Input: part model. Units: mm. Frame: model coordinates. Face numbers are marked on the shaded views. A direction names the side the tool comes from. Give positions to 0.01 mm unless a question says otherwise; leave off trailing zeros. Write each loop counter-clockwise with the first axis right and the second up, starting at its lowest first coordinate (ties: lowest second). Pieces come first, ordered by that corner, then holes. Notation, with made-up numbers: (55.5, -6.5) -> (100.5, -6.5) arc R29 cw to (100.5, 15.5) -> close; hole circle Ø5 at (-28, 54). An arc over 180 degrees is marked (long way). Return JSON: item names as keys, results as strings. Group by question number.
Item 1: Mould query, pull axis X, two halves, no side actions, for the marked faces 4, 5, 6 and 7. Classes: released by +X, released by -X, zero draft, split by the parting line, or undercut.
Item 2: Section D-D, the plane y = 21.5. Return loops of the section in (x, z).
Item 3: Pin query (flat end, axial travel): P1, Ø3, axis at x = 88, y = 47.5, coming from the +Z side; P2, Ø4, axis at x = 31.5, y = 11, coming from the +Z side. Return the tip coordinate at first contact, or that it passes through.
Item 4: Section B-B, the plane z = 8.5. Return loops of the section in (x, y).
Item 5: Section A-A, the plane y = 81.75. Return loops of the section in (x, z).
Item 6: Line query: line 1 (Y direction, x = 139.5, z = 19.5); line 2 (X direction, y = 5.75, z = 26); line 3 (Z direction, x = 146, y = 36). Output: solid intervals per line, ascending. Write a range as [from, to].
Item 7: Set-up query: the marked faces 1, 2 and 3. Return all of +Z, -Z, +X, -X, +Y, -Y with unobstructed straight access to the full face (end or side cutting, diameter ignored); none if empty.
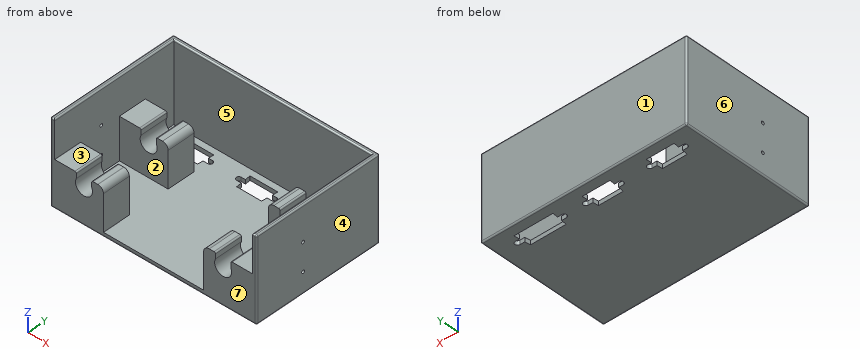
from build123d import *

# Parameters (mm, degrees)
CYLINDER009_R      = 1.1
CYLINDER009_DEPTH  = 150
CYLINDER008_R      = 1.1
CYLINDER008_DEPTH  = 150
BOX011_W           = 25.4
BOX011_H           = 3.6
BOX011_DEPTH       = 10
CYLINDER005_R      = 1.8
CYLINDER005_DEPTH  = 10
CYLINDER004_R      = 1.8
CYLINDER004_DEPTH  = 10
BOX010_W           = 20
BOX010_H           = 11.5
BOX010_DEPTH       = 10
CHAMFER001_1_SIZE2 = 1.1
CHAMFER001_1_SIZE  = 11
CHAMFER001_2_SIZE2 = 1.1
CHAMFER001_2_SIZE  = 11
BOX013_W           = 25.4
BOX013_H           = 3.6
BOX013_DEPTH       = 10
CYLINDER006_R      = 1.8
CYLINDER006_DEPTH  = 10
CYLINDER007_R      = 1.8
CYLINDER007_DEPTH  = 10
BOX012_W           = 20
BOX012_H           = 11.5
BOX012_DEPTH       = 10
CHAMFER002_1_SIZE2 = 1.1
CHAMFER002_1_SIZE  = 11
CHAMFER002_2_SIZE2 = 1.1
CHAMFER002_2_SIZE  = 11
CYLINDER003_R      = 1.8
CYLINDER003_DEPTH  = 10
BOX009_W           = 33.6
BOX009_H           = 3.6
BOX009_DEPTH       = 10
CYLINDER002_R      = 1.8
CYLINDER002_DEPTH  = 10
BOX008_W           = 28
BOX008_H           = 11.5
BOX008_DEPTH       = 10
CHAMFER_1_SIZE2    = 1.2
CHAMFER_1_SIZE     = 11
CHAMFER_2_SIZE2    = 1.2
CHAMFER_2_SIZE     = 11
BOX006_W           = 11
BOX006_H           = 73
BOX006_DEPTH       = 15
BOX007_W           = 11
BOX007_H           = 73
BOX007_DEPTH       = 15
CYLINDER001_R      = 6.1
CYLINDER001_DEPTH  = 80
CYLINDER_R         = 6.1
CYLINDER_DEPTH     = 80
BOX002_W           = 35
BOX002_H           = 20
BOX002_DEPTH       = 30
BOX003_W           = 35
BOX003_H           = 20
BOX003_DEPTH       = 30
BOX004_W           = 35
BOX004_H           = 20
BOX004_DEPTH       = 30
BOX005_W           = 35
BOX005_H           = 20
BOX005_DEPTH       = 30
BOX001_W           = 142
BOX001_H           = 92
BOX001_DEPTH       = 60
BOX_W              = 148
BOX_H              = 95
BOX_DEPTH          = 60
FILLET_R           = 1
FILLET001_R        = 4
FILLET002_R        = 1


with BuildPart() as cylinder009:
    # Cylinder009 → Cylinder009 (new body)
    with BuildSketch(Plane(origin=(-1, 36, 35), x_dir=(0, 0, -1), z_dir=(1, 0, 0))):
        Circle(CYLINDER009_R)
    extrude(amount=CYLINDER009_DEPTH)


with BuildPart() as cylinder008:
    # Cylinder008 → Cylinder008 (new body)
    with BuildSketch(Plane(origin=(-1, 36, 15), x_dir=(0, 0, -1), z_dir=(1, 0, 0))):
        Circle(CYLINDER008_R)
    extrude(amount=CYLINDER008_DEPTH)


with BuildPart() as cube011:
    # Box011 → Box011 (new body)
    with BuildSketch(Plane(origin=(-2.7, 3.95, 0), x_dir=(1, 0, 0), z_dir=(0, 0, 1))):
        with Locations((12.7, 1.8)):
            Rectangle(BOX011_W, BOX011_H)
    extrude(amount=BOX011_DEPTH)


with BuildPart() as cylinder005:
    # Cylinder005 → Cylinder005 (new body)
    with BuildSketch(Plane(origin=(22.7, 5.75, 0), x_dir=(1, 0, 0), z_dir=(0, 0, 1))):
        Circle(CYLINDER005_R)
    extrude(amount=CYLINDER005_DEPTH)


with BuildPart() as cylinder004:
    # Cylinder004 → Cylinder004 (new body)
    with BuildSketch(Plane(origin=(-2.7, 5.75, 0), x_dir=(1, 0, 0), z_dir=(0, 0, 1))):
        Circle(CYLINDER004_R)
    extrude(amount=CYLINDER004_DEPTH)


with BuildPart() as obj1:
    # Box010 → Box010 (new body)
    with BuildSketch(Plane.XY):
        with Locations((10, 5.75)):
            Rectangle(BOX010_W, BOX010_H)
    extrude(amount=BOX010_DEPTH)

    # Chamfer001 1
    chamfer001_1_edges = [obj1.edges().sort_by_distance(p)[0] for p in [
        (20, 0, 5),
    ]]
    chamfer001_1_side = obj1.faces().sort_by_distance((20, 5.75, 5))[0]
    chamfer(chamfer001_1_edges, length=CHAMFER001_1_SIZE, length2=CHAMFER001_1_SIZE2, reference=chamfer001_1_side)

    # Chamfer001 2
    chamfer001_2_edges = [obj1.edges().sort_by_distance(p)[0] for p in [
        (0, 0, 5),
    ]]
    chamfer001_2_side = obj1.faces().sort_by_distance((0, 5.75, 5))[0]
    chamfer(chamfer001_2_edges, length=CHAMFER001_2_SIZE, length2=CHAMFER001_2_SIZE2, reference=chamfer001_2_side)

    # Fusion002: union Cube011, Cylinder005, Cylinder004
    add(cube011.part)
    add(cylinder005.part)
    add(cylinder004.part)


with BuildPart() as obj1_1:
    # Fusion002 placement: moved
    add(obj1.part.moved(Location((16, 76, 0))))


with BuildPart() as cube013:
    # Box013 → Box013 (new body)
    with BuildSketch(Plane(origin=(-2.7, 3.95, 0), x_dir=(1, 0, 0), z_dir=(0, 0, 1))):
        with Locations((12.7, 1.8)):
            Rectangle(BOX013_W, BOX013_H)
    extrude(amount=BOX013_DEPTH)


with BuildPart() as cylinder006:
    # Cylinder006 → Cylinder006 (new body)
    with BuildSketch(Plane(origin=(22.7, 5.75, 0), x_dir=(1, 0, 0), z_dir=(0, 0, 1))):
        Circle(CYLINDER006_R)
    extrude(amount=CYLINDER006_DEPTH)


with BuildPart() as cylinder007:
    # Cylinder007 → Cylinder007 (new body)
    with BuildSketch(Plane(origin=(-2.7, 5.75, 0), x_dir=(1, 0, 0), z_dir=(0, 0, 1))):
        Circle(CYLINDER007_R)
    extrude(amount=CYLINDER007_DEPTH)


with BuildPart() as obj2:
    # Box012 → Box012 (new body)
    with BuildSketch(Plane.XY):
        with Locations((10, 5.75)):
            Rectangle(BOX012_W, BOX012_H)
    extrude(amount=BOX012_DEPTH)

    # Chamfer002 1
    chamfer002_1_edges = [obj2.edges().sort_by_distance(p)[0] for p in [
        (20, 0, 5),
    ]]
    chamfer002_1_side = obj2.faces().sort_by_distance((20, 5.75, 5))[0]
    chamfer(chamfer002_1_edges, length=CHAMFER002_1_SIZE, length2=CHAMFER002_1_SIZE2, reference=chamfer002_1_side)

    # Chamfer002 2
    chamfer002_2_edges = [obj2.edges().sort_by_distance(p)[0] for p in [
        (0, 0, 5),
    ]]
    chamfer002_2_side = obj2.faces().sort_by_distance((0, 5.75, 5))[0]
    chamfer(chamfer002_2_edges, length=CHAMFER002_2_SIZE, length2=CHAMFER002_2_SIZE2, reference=chamfer002_2_side)

    # Fusion003: union Cube013, Cylinder006, Cylinder007
    add(cube013.part)
    add(cylinder006.part)
    add(cylinder007.part)


with BuildPart() as obj2_1:
    # Fusion003 placement: moved
    add(obj2.part.moved(Location((62, 76, 0))))


with BuildPart() as cylinder003:
    # Cylinder003 → Cylinder003 (new body)
    with BuildSketch(Plane(origin=(30.8, 5.75, 0), x_dir=(1, 0, 0), z_dir=(0, 0, 1))):
        Circle(CYLINDER003_R)
    extrude(amount=CYLINDER003_DEPTH)


with BuildPart() as cube009:
    # Box009 → Box009 (new body)
    with BuildSketch(Plane(origin=(-2.8, 3.95, 0), x_dir=(1, 0, 0), z_dir=(0, 0, 1))):
        with Locations((16.8, 1.8)):
            Rectangle(BOX009_W, BOX009_H)
    extrude(amount=BOX009_DEPTH)


with BuildPart() as cylinder002:
    # Cylinder002 → Cylinder002 (new body)
    with BuildSketch(Plane(origin=(-2.8, 5.75, 0), x_dir=(1, 0, 0), z_dir=(0, 0, 1))):
        Circle(CYLINDER002_R)
    extrude(amount=CYLINDER002_DEPTH)


with BuildPart() as obj3:
    # Box008 → Box008 (new body)
    with BuildSketch(Plane.XY):
        with Locations((14, 5.75)):
            Rectangle(BOX008_W, BOX008_H)
    extrude(amount=BOX008_DEPTH)

    # Chamfer 1
    chamfer_1_edges = [obj3.edges().sort_by_distance(p)[0] for p in [
        (28, 0, 5),
    ]]
    chamfer_1_side = obj3.faces().sort_by_distance((28, 5.75, 5))[0]
    chamfer(chamfer_1_edges, length=CHAMFER_1_SIZE, length2=CHAMFER_1_SIZE2, reference=chamfer_1_side)

    # Chamfer 2
    chamfer_2_edges = [obj3.edges().sort_by_distance(p)[0] for p in [
        (0, 0, 5),
    ]]
    chamfer_2_side = obj3.faces().sort_by_distance((0, 5.75, 5))[0]
    chamfer(chamfer_2_edges, length=CHAMFER_2_SIZE, length2=CHAMFER_2_SIZE2, reference=chamfer_2_side)

    # Fusion001: union Cylinder003, Cube009, Cylinder002
    add(cylinder003.part)
    add(cube009.part)
    add(cylinder002.part)


with BuildPart() as obj3_1:
    # Fusion001 placement: moved
    add(obj3.part.moved(Location((103, 76, 0))))


with BuildPart() as cube006:
    # Box006 → Box006 (new body)
    with BuildSketch(Plane(origin=(118.5, 0, 27), x_dir=(1, 0, 0), z_dir=(0, 0, 1))):
        with Locations((5.5, 36.5)):
            Rectangle(BOX006_W, BOX006_H)
    extrude(amount=BOX006_DEPTH)


with BuildPart() as cube007:
    # Box007 → Box007 (new body)
    with BuildSketch(Plane(origin=(18.5, 0, 27), x_dir=(1, 0, 0), z_dir=(0, 0, 1))):
        with Locations((5.5, 36.5)):
            Rectangle(BOX007_W, BOX007_H)
    extrude(amount=BOX007_DEPTH)


with BuildPart() as cylinder001:
    # Cylinder001 → Cylinder001 (new body)
    with BuildSketch(Plane(origin=(124, 73, 26), x_dir=(1, 0, 0), z_dir=(0, -1, 0))):
        Circle(CYLINDER001_R)
    extrude(amount=CYLINDER001_DEPTH)


with BuildPart() as cylinder:
    # Cylinder → Cylinder (new body)
    with BuildSketch(Plane(origin=(24, 73, 26), x_dir=(1, 0, 0), z_dir=(0, -1, 0))):
        Circle(CYLINDER_R)
    extrude(amount=CYLINDER_DEPTH)


with BuildPart() as cube002:
    # Box002 → Box002 (new body)
    with BuildSketch(Plane(origin=(3, 0, 3), x_dir=(1, 0, 0), z_dir=(0, 0, 1))):
        with Locations((17.5, 10)):
            Rectangle(BOX002_W, BOX002_H)
    extrude(amount=BOX002_DEPTH)


with BuildPart() as cube003:
    # Box003 → Box003 (new body)
    with BuildSketch(Plane(origin=(3, 50, 3), x_dir=(1, 0, 0), z_dir=(0, 0, 1))):
        with Locations((17.5, 10)):
            Rectangle(BOX003_W, BOX003_H)
    extrude(amount=BOX003_DEPTH)


with BuildPart() as cube004:
    # Box004 → Box004 (new body)
    with BuildSketch(Plane(origin=(110, 0, 3), x_dir=(1, 0, 0), z_dir=(0, 0, 1))):
        with Locations((17.5, 10)):
            Rectangle(BOX004_W, BOX004_H)
    extrude(amount=BOX004_DEPTH)


with BuildPart() as cube005:
    # Box005 → Box005 (new body)
    with BuildSketch(Plane(origin=(110, 50, 3), x_dir=(1, 0, 0), z_dir=(0, 0, 1))):
        with Locations((17.5, 10)):
            Rectangle(BOX005_W, BOX005_H)
    extrude(amount=BOX005_DEPTH)


with BuildPart() as cube001:
    # Box001 → Box001 (new body)
    with BuildSketch(Plane(origin=(3, 0, 3), x_dir=(1, 0, 0), z_dir=(0, 0, 1))):
        with Locations((71, 46)):
            Rectangle(BOX001_W, BOX001_H)
    extrude(amount=BOX001_DEPTH)


with BuildPart() as fillet002:
    # Box → Box (new body)
    with BuildSketch(Plane.XY):
        with Locations((74, 47.5)):
            Rectangle(BOX_W, BOX_H)
    extrude(amount=BOX_DEPTH)

    # Cut: cut Cube001
    add(cube001.part, mode=Mode.SUBTRACT)

    # Fusion: union Cube002, Cube003, Cube004, Cube005
    add(cube002.part)
    add(cube003.part)
    add(cube004.part)
    add(cube005.part)

    # Cut001: cut Cylinder
    add(cylinder.part, mode=Mode.SUBTRACT)

    # Cut002: cut Cylinder001
    add(cylinder001.part, mode=Mode.SUBTRACT)

    # Cut003: cut Cube007
    add(cube007.part, mode=Mode.SUBTRACT)

    # Cut004: cut Cube006
    add(cube006.part, mode=Mode.SUBTRACT)

    # Fillet
    fillet_edges = [fillet002.edges().sort_by_distance(p)[0] for p in [
        (29.5, 10, 33),
        (18.5, 10, 33),
        (18.5, 60, 33),
        (29.5, 60, 33),
        (129.5, 60, 33),
        (129.5, 10, 33),
        (118.5, 60, 33),
        (118.5, 10, 33),
    ]]
    fillet(fillet_edges, radius=FILLET_R)

    # Fillet001
    fillet001_edges = [fillet002.edges().sort_by_distance(p)[0] for p in [
        (38, 10, 33),
        (38, 60, 33),
        (110, 60, 33),
        (110, 10, 33),
    ]]
    fillet(fillet001_edges, radius=FILLET001_R)

    # Cut005: cut obj3
    add(obj3_1.part, mode=Mode.SUBTRACT)

    # Cut006: cut obj2
    add(obj2_1.part, mode=Mode.SUBTRACT)

    # Cut007: cut obj1
    add(obj1_1.part, mode=Mode.SUBTRACT)

    # Cut008: cut Cylinder008
    add(cylinder008.part, mode=Mode.SUBTRACT)

    # Cut009: cut Cylinder009
    add(cylinder009.part, mode=Mode.SUBTRACT)

    # Fillet002
    fillet002_edges = [fillet002.edges().sort_by_distance(p)[0] for p in [
        (148, 0, 30),
        (146.5, 0, 60),
        (1.5, 0, 60),
        (0, 0, 30),
        (74, 0, 0),
        (148, 47.5, 60),
        (148, 47.5, 0),
        (148, 95, 30),
        (74, 95, 60),
        (145, 46, 60),
        (74, 92, 60),
        (3, 46, 60),
        (0, 47.5, 60),
        (0, 47.5, 0),
        (0, 95, 30),
        (74, 95, 0),
    ]]
    fillet(fillet002_edges, radius=FILLET002_R)


solid = fillet002.part
Answer below:
{
 "1": {"face 4": "released by +X", "face 5": "undercut", "face 6": "released by -X", "face 7": "zero draft"},
 "2": {"outline": "(0, 1) arc R1 ccw to (1, 0) -> (147, 0) arc R1 ccw to (148, 1) -> (148, 59) arc R1 ccw to (147, 60) -> (146, 60) arc R1 ccw to (145, 59) -> (145, 3) -> (3, 3) -> (3, 59) arc R1 ccw to (2, 60) -> (1, 60) arc R1 ccw to (0, 59) -> close"},
 "3": {"P1": "stops at z = 3", "P2": "stops at z = 33"},
 "4": {"outline": "(0, 1) arc R1 ccw to (1, 0) -> (38, 0) -> (38, 20) -> (3, 20) -> (3, 50) -> (38, 50) -> (38, 70) -> (3, 70) -> (3, 92) -> (145, 92) -> (145, 70) -> (110, 70) -> (110, 50) -> (145, 50) -> (145, 20) -> (110, 20) -> (110, 0) -> (147, 0) arc R1 ccw to (148, 1) -> (148, 94) arc R1 ccw to (147, 95) -> (1, 95) arc R1 ccw to (0, 94) -> close"},
 "5": {"outline": "(0, 1) arc R1 ccw to (1, 0) -> (11.5, 0) -> (11.5, 3) -> (3, 3) -> (3, 59) arc R1 ccw to (2, 60) -> (1, 60) arc R1 ccw to (0, 59) -> close; (40.5, 0) -> (57.5, 0) -> (57.5, 3) -> (40.5, 3) -> close; (86.5, 0) -> (98.4, 0) -> (98.4, 3) -> (86.5, 3) -> close; (135.6, 0) -> (147, 0) arc R1 ccw to (148, 1) -> (148, 59) arc R1 ccw to (147, 60) -> (146, 60) arc R1 ccw to (145, 59) -> (145, 3) -> (135.6, 3) -> close"},
 "6": {"line 1": "y = [0, 20], [50, 70], [92, 95]", "line 2": "x = [0, 17.9], [30.1, 38], [110, 117.9], [130.1, 148]", "line 3": "z = [0, 13.9], [16.1, 33.9], [36.1, 60]"},
 "7": {"face 1": "+Z, -Z, +X, -X, +Y", "face 2": "+Z", "face 3": "+Z, -Y"}
}
